The model under review builds one solid part; all positions refer to its coordinate system, in mm. Face numbers are marked on the shaded views. A direction names the side the tool comes from. Coordinates: 2 decimals unless noted, no trailing zeros. Loops run counter-clockwise (first coordinate to the right, second up) from the corner with the lowest first, then second, coordinate; pieces in that order, holes last. Notation, with made-up numbers: M -24,80 L -16,80 A24 cw -16,108 Z; hole C -14.5,52.25 d1. An arc over 180 degrees is marked long. Use CSV: the item, a comma, the result in double quotes. Start each with the question number.
from build123d import *

# Parameters (mm, degrees)
SKETCH_1_R                = 85
SKETCH_1_R_2              = 4
SKETCH_1_R_3              = 3
EXTRUDE_1_DEPTH           = 18
HOLE_WIZARD_1_D           = 6.6
HOLE_WIZARD_1_CBORE_D     = 11
HOLE_WIZARD_1_CBORE_DEPTH = 6.8
HOLE_WIZARD_M8_1_D        = 6.8
SKETCH_6_R                = 15
EXTRUDE_2_DEPTH           = 32


with BuildPart() as part:
    # 草图1 → 凸台-拉伸1 (new body)
    with BuildSketch(Plane.XY):
        Circle(SKETCH_1_R)
        with Locations((0, 77.5)):
            Circle(SKETCH_1_R_2, mode=Mode.SUBTRACT)
        with Locations((67.116968793, 38.75)):
            Circle(SKETCH_1_R_2, mode=Mode.SUBTRACT)
        with Locations((67.116968793, -38.75)):
            Circle(SKETCH_1_R_2, mode=Mode.SUBTRACT)
        with Locations((0, -77.5)):
            Circle(SKETCH_1_R_2, mode=Mode.SUBTRACT)
        with Locations((-67.116968793, -38.75)):
            Circle(SKETCH_1_R_2, mode=Mode.SUBTRACT)
        with Locations((-67.116968793, 38.75)):
            Circle(SKETCH_1_R_2, mode=Mode.SUBTRACT)
        with Locations((-14.849242405, 14.849242405)):
            Circle(SKETCH_1_R_3, mode=Mode.SUBTRACT)
        with Locations((14.849242405, 14.849242405)):
            Circle(SKETCH_1_R_3, mode=Mode.SUBTRACT)
        with Locations((14.849242405, -14.849242405)):
            Circle(SKETCH_1_R_3, mode=Mode.SUBTRACT)
        with Locations((-14.849242405, -14.849242405)):
            Circle(SKETCH_1_R_3, mode=Mode.SUBTRACT)
    extrude(amount=EXTRUDE_1_DEPTH)

    # 打孔尺寸(%根据)内六角圆柱头螺钉的类型1 (through all)
    with Locations(Plane.XY.offset(18)):
        with Locations((-67.116968793, 38.75), (67.116968793, 38.75), (67.116968793, -38.75), (-67.116968793, -38.75)):
            CounterBoreHole(HOLE_WIZARD_1_D / 2, HOLE_WIZARD_1_CBORE_D / 2, HOLE_WIZARD_1_CBORE_DEPTH)

    # M8 螺纹孔1 (through all)
    with Locations(Plane.XY.offset(18)):
        with Locations((-14.849242405, 14.849242405), (14.849242405, 14.849242405), (14.849242405, -14.849242405), (-14.849242405, -14.849242405)):
            Hole(HOLE_WIZARD_M8_1_D / 2)

    # 草图6 → 凸台-拉伸2 (add)
    with BuildSketch(Plane.XY.offset(18)):
        Circle(SKETCH_6_R)
    extrude(amount=EXTRUDE_2_DEPTH)


solid = part.part
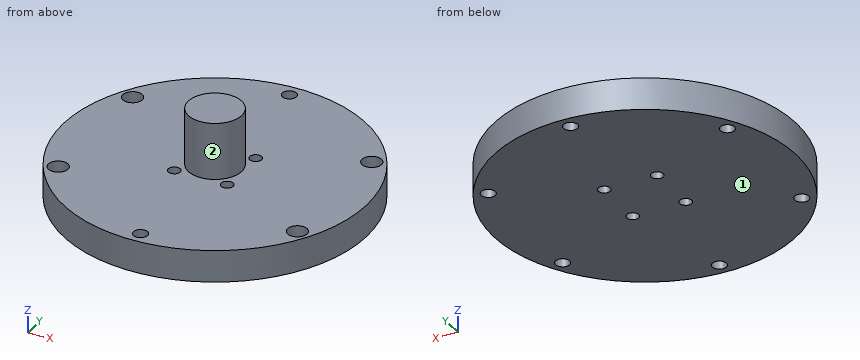
1. Add section C-C (z = 42.5). Write out the cut boundary in (x, y).
2. Add section B-B (y = -77.5). Write out the cut boundary in (x, z), plus the area to 3 significant figures.
3. Insertion check: pin 1 Ø3 at (x, y) = (63.5, -4.5) entering from +Z; pin 2 Ø5.5 at (x, y) = (66.5, 41) entering from +Z; pin 3 Ø5 at (x, z) = (-0.5, 23.5) entering from +Y. Each pin has a flat end and moves straight along its axis. Give the tip position at first contact, or say it passes through.
4. For the marked faces 1 and 2, list the 3-axis set-ups (+Z, -Z, +X, -X, +Y, -Y) from which the entire face can be reached by the end or side of a thin tool; tool diameter is ignored.
5. Add section D-D (y = 8.5). Write out the cut boundary in (x, z).
6. Add section A-A (y = -38.75). Write out the cut boundary in (x, z), plus the area to 3 significant figures.
7. To check wall thickness, follow line 1 along Y through (x, z) = (-64, 16); line 2 along Z through (x, y) = (54, -19.5); line 3 along X through (y, z) = (-38.75, 7.75). State the ranges of each line that lie inside material, in increasing order.
Solved:
1,outline,"C 0,0 d30"
2,outline,"M -34.91,0 L -4,0 L -4,18 L -34.91,18 Z; M 4,0 L 34.91,0 L 34.91,18 L 4,18 Z"
2,area,"1,110 mm^2"
3,pin 1,"stops at z = 18"
3,pin 2,"stops at z = 11.2"
3,pin 3,"stops at y = 15"
4,face 1,"-Z, +X, -X, +Y, -Y"
4,face 2,"+Z"
5,outline,"M -84.57,0 L 84.57,0 L 84.57,18 L 12.36,18 L 12.36,50 L -12.36,50 L -12.36,18 L -84.57,18 Z"
6,outline,"M -75.65,0 L -71.12,0 L -71.12,11.2 L -72.62,11.2 L -72.62,18 L -75.65,18 Z; M -63.12,0 L 63.12,0 L 63.12,11.2 L 61.62,11.2 L 61.62,18 L -61.62,18 L -61.62,11.2 L -63.12,11.2 Z; M 71.12,0 L 75.65,0 L 75.65,18 L 72.62,18 L 72.62,11.2 L 71.12,11.2 Z"
6,area,"2,390 mm^2"
7,line 1,"y = -55.94 to -43.28, -34.22 to 34.22, 43.28 to 55.94"
7,line 2,"z = 0 to 18"
7,line 3,"x = -75.65 to -71.12, -63.12 to 63.12, 71.12 to 75.65"
